Could you check a few things on this model? Use its own coordinates, in mm. Coordinates: 2 decimals unless noted, no trailing zeros. Loops run counter-clockwise (first coordinate to the right, second up) from the corner with the lowest first, then second, coordinate; pieces in that order, holes last. Notation, with made-up numbers: M -30.5,68 L -3.5,68 A27 cw -3.5,97 Z; hole C 57,41 d5. An arc over 180 degrees is marked long. Return JSON: item names as keys, results as strings. Group by question number.
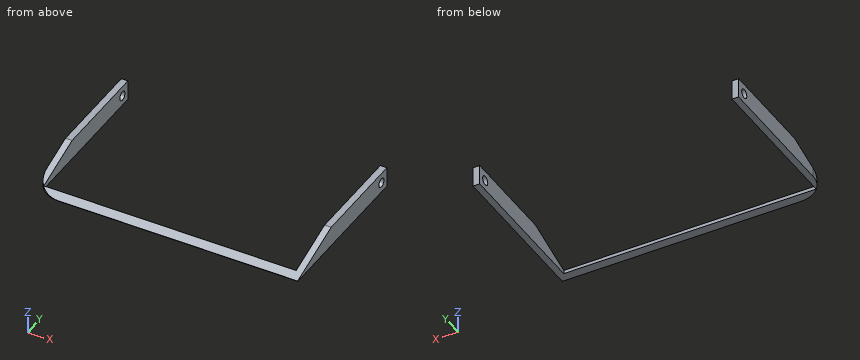
from build123d import *

# Parameters (mm, degrees)
F0_W     = 200
F0_H     = 120
F1_DEPTH = 15
F2_R     = 3.4108766744
F3_DEPTH = 200.001
F4_SIZE2 = 14.75
F4_SIZE  = 45
F5_R     = 20
F6_W     = 190
F6_H     = 113
F7_DEPTH = 15.001


with BuildPart() as f1:
    # F0 (on Top) → F1 (new body)
    with BuildSketch(Plane.XY):
        Rectangle(F0_W, F0_H)
    extrude(amount=F1_DEPTH)

    # F2 (on face) → F3 (cut, through all)
    with BuildSketch(Plane.YZ.offset(100)):
        with Locations((52.5, 7.5)):
            Circle(F2_R)
    extrude(amount=-F3_DEPTH, mode=Mode.SUBTRACT)

    # F4
    f4_edges = [f1.edges().sort_by_distance(p)[0] for p in [
        (0, -60, 15),
    ]]
    f4_side = f1.faces().sort_by_distance((0, 0, 15))[0]
    chamfer(f4_edges, length=F4_SIZE, length2=F4_SIZE2, reference=f4_side)

    # F5
    f5_edges = [f1.edges().sort_by_distance(p)[0] for p in [
        (-100, -60, 0.125),
    ]]
    fillet(f5_edges, radius=F5_R)

    # F6 (on face) → F7 (cut, through all)
    with BuildSketch(Plane.XY.offset(15)):
        with Locations((0, 3.5)):
            Rectangle(F6_W, F6_H)
    extrude(amount=-F7_DEPTH, mode=Mode.SUBTRACT)


solid = f1.part
(1) Imagine slicing it at C-C, the plane x = -4.5. Write out the boundary of the cut face in (y, z).
(2) Imagine slicing it at B-B, the plane y = 52.5. Write out the boundary of the cut face in (x, z), then the cut area to 3 significant figures.
(3) Will this pin go through, and if not, where does the flat tip stop? P1, Ø2, axis at x = 24, z = 1, coming from the +Y side.
(4) If I drill on L1, parallel to X at y = 35.5, z = 10.5; L2, parallel to Z at x = -98.8, y = 52.5; L3, parallel to X at y = -46, z = 2.5, over which ranges is the centre line in solid material (lowest first)? Write a range as [from, to].
(5) Imagine slicing it at D-D, the plane x = -84.5. Write out the boundary of the cut face in (y, z), then the cut area to 3 significant figures.
(6) Imagine slicing it at A-A, the plane y = 30. Write out the boundary of the cut face in (x, z).
Checks:
{
 "1": {"outline": "M -60,0 L -53,0 L -53,2.54 L -60,0.25 Z"},
 "2": {"outline": "M -100,0 L -95,0 L -95,4.09 L -100,4.09 Z; M -100,10.91 L -95,10.91 L -95,15 L -100,15 Z; M 95,0 L 100,0 L 100,4.09 L 95,4.09 Z; M 95,10.91 L 100,10.91 L 100,15 L 95,15 Z", "area": "81.8 mm²"},
 "3": {"P1": "y = -53"},
 "4": {"L1": "[-100, -95], [95, 100]", "L2": "[0, 4.09], [10.91, 15]", "L3": "[-99.08, -95], [95, 100]"},
 "5": {"outline": "M -59.49,0 L -53,0 L -53,2.54 L -59.49,0.42 Z", "area": "9.61 mm²"},
 "6": {"outline": "M -100,0 L -95,0 L -95,15 L -100,15 Z; M 95,0 L 100,0 L 100,15 L 95,15 Z"}
}
